from build123d import *

# Parameters (mm, degrees)
CROQUIS1_R              = 5.55
CROQUIS1_R_2            = 1.45
SALIENTE_EXTRUIR1_DEPTH = 7
CHAFL_N1_SIZE           = 1.5
CROQUIS2_R              = 8
CROQUIS2_R_2            = 5.55
SALIENTE_EXTRUIR2_DEPTH = 3
CHAFL_N2_SIZE           = 2.5


with BuildPart() as part:
    # Croquis1 → Saliente-Extruir1 (new body)
    with BuildSketch(Plane.XY):
        Circle(CROQUIS1_R)
        Circle(CROQUIS1_R_2, mode=Mode.SUBTRACT)
    extrude(amount=SALIENTE_EXTRUIR1_DEPTH)

    # Chaflán1
    chafl_n1_edges = [part.edges().sort_by_distance(p)[0] for p in [
        (-1.45, 0, 7),
    ]]
    chamfer(chafl_n1_edges, length=CHAFL_N1_SIZE)

    # Croquis2 → Saliente-Extruir2 (add)
    with BuildSketch(Plane.XY.offset(4)):
        Circle(CROQUIS2_R)
        Circle(CROQUIS2_R_2, mode=Mode.SUBTRACT)
    extrude(amount=SALIENTE_EXTRUIR2_DEPTH)

    # Chaflán2
    chafl_n2_edges = [part.edges().sort_by_distance(p)[0] for p in [
        (-8, 0, 7),
    ]]
    chamfer(chafl_n2_edges, length=CHAFL_N2_SIZE)


solid = part.part
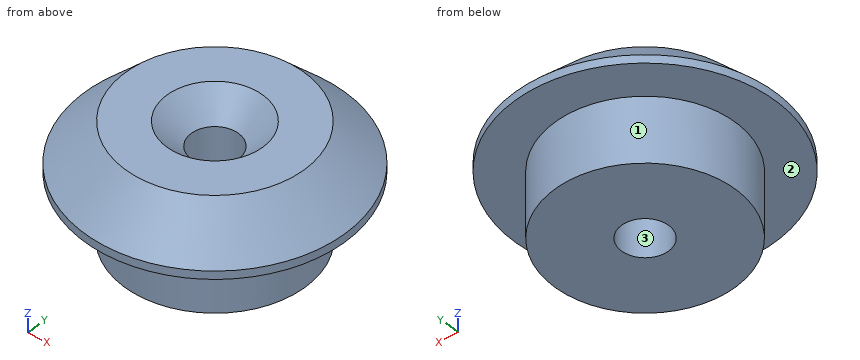
Here's how the part is built. I have some questions about the finished solid (model axes, mm). Face numbers are marked on the shaded views. Coordinates: 2 decimals unless noted, no trailing zeros. Write each loop counter-clockwise with the first axis right and the second up, starting at its lowest first coordinate (ties: lowest second). Pieces come first, ordered by that corner, then holes.
Item 1: I want a section at A-A on y = 0. Write out the boundary of the cut face in (x, z).
Item 2: If we mould it in two halves opening along Y, with no side actions, what happens to the marked faces 1, 2 and 3? For each: +Y half, -Y half, draft (parallel to the pull), parting line (faces both ways), or undercut.
Item 3: I want a section at D-D on z = 1.25. Write out the boundary of the cut face in (x, y), and give its area (3 significant figures).
Item 4: I want a section at C-C on z = 5. Write out the boundary of the cut face in (x, y), and give its area (3 significant figures).
Item 5: If I drill on line 1 (Y direction, x = 0, z = 3); line 2 (Y direction, x = 0.5, z = 5); line 3 (Z direction, x = -2, y = 5.5), over which ranges is the centre line in solid material (lowest first)?
Item 6: Will these pins go through, and if not, where does the flat tip stop? pin 1 (1.5 mm diameter, centred on x = -4, z = 4.5, fed in from +Y); pin 2 (4.5 mm diameter, centred on x = 0, y = 0, fed in from -Z); pin 3 (1 mm diameter, centred on x = 4, z = 4.5, fed in from +Y); pin 4 (2 mm diameter, centred on x = -1, y = 0, fed in from +Z).
Findings below:
1. outline: (-8, 4) - (-5.55, 4) - (-5.55, 0) - (-1.45, 0) - (-1.45, 5.5) - (-2.95, 7) - (-5.5, 7) - (-8, 4.5) - close; (1.45, 0) - (5.55, 0) - (5.55, 4) - (8, 4) - (8, 4.5) - (5.5, 7) - (2.95, 7) - (1.45, 5.5) - close
2. face 1: parting line
2. face 2: draft
2. face 3: undercut
3. outline: circle Ø11.1 at (0, 0); hole circle Ø2.9 at (0, 0)
3. area: 90.2 mm2
4. outline: circle Ø15 at (0, 0); hole circle Ø2.9 at (0, 0)
4. area: 170 mm2
5. line 1: y = -5.55 to -1.45, 1.45 to 5.55
5. line 2: y = -7.48 to -1.36, 1.36 to 7.48
5. line 3: z = 4 to 6.65
6. pin 1: stops at y = 7.31
6. pin 2: stops at z = 0
6. pin 3: stops at y = 7.19
6. pin 4: stops at z = 6.05
